The listing builds one solid part. Answer for the finished solid, in the listing's coordinates (mm). Face numbers are marked on the shaded views. A direction names the side the tool comes from. Round coordinates to 2 decimals unless told otherwise and drop trailing zeros. Order: outer loops, then holes, each group sorted by start corner. A loop starts at its lowest first (then second) coordinate and runs counter-clockwise, first axis right, second up. Notation, with made-up numbers: M 22,79.25 L 58,79.25 A27 cw 58,115.25 Z; hole C 82,-18.5 d3. An arc over 180 degrees is marked long. Write item = value, one per line. Start each with the question number.
(1) A cutting plane is placed at C-C, the plane z = 0. Determine the outline of the cut face in (x, y).
(2) A cutting plane is placed at B-B, the plane x = -14.5. Determine the outline of the cut face in (y, z), and give its area (3 significant figures).
(3) Each of these flat-tipped pins is pushed along its axis until it touches: pin 1 (1 mm diameter, centred on y = 17, z = -20, fed in from -X); pin 2 (4.5 mm diameter, centred on y = 8.69, z = -18.47, fed in from +X); pin 3 (3 mm diameter, centred on x = -17.5, y = 7, fed in from +Z). Where does it stop, or does it pass through?
(4) A cutting plane is placed at A-A, the plane z = -18. Determine the outline of the cut face in (x, y), and give its area (3 significant figures).
(5) Which of the six approach directions +Z, -Z, +X, -X, +Y, -Y give full straight-line access (tool end or side, diameter ignored) to the marked faces 4, 5, 6, 7 and 8?
(6) Straight lines are drawn through the part: probe 1 along X at (y, z) = (12.5, -13); probe 2 along X at (y, z) = (14.25, 15); probe 3 along Z at (x, y) = (0, 20). For each, find the intervals that lie inside material, in ascending order. Write a range as from..to.
(7) A cutting plane is placed at D-D, the plane x = 12.5. Determine the outline of the cut face in (y, z), and give its area (3 significant figures).
(8) For a pull along X with two mould halves and no side action, classify the marked faces 1, 2 and 3 as released by +X, released by -X, zero draft, split by the parting line, or undercut.
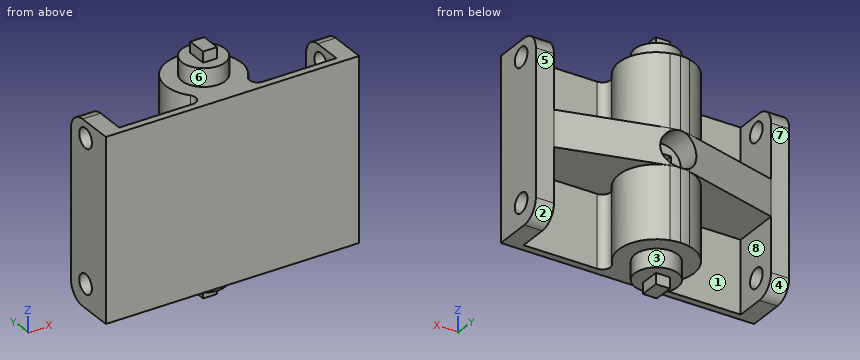
from build123d import *
from build123d.topology import SkipClean

# Parameters (mm, degrees)
BOSS_EXTRUDE1_DEPTH      = 5
BOSS_EXTRUDE2_DEPTH      = 20
MIRROR3_COPY_1_DEPTH     = 5
MIRROR3_COPY_2_DEPTH     = 20
SKETCH4_R                = 2.698355907
CUT_EXTRUDE1_DEPTH       = 5
BOSS_EXTRUDE3_DEPTH      = 5
BOSS_EXTRUDE3_DEPTH_BACK = 55
SKETCH8_R                = 5.951026126
SKETCH8_W                = 3.866122338
SKETCH8_H                = 5.532358837
BOSS_EXTRUDE5_DEPTH      = 3
BOSS_EXTRUDE5_DEPTH_BACK = 63
SKETCH10_W               = 3.866122338
SKETCH10_H               = 5.532358837
SKETCH12_R               = 5
CUT_EXTRUDE3_DEPTH       = 7.59683428
SKETCH14_W               = 4.609426796
SKETCH14_H               = 4.865506062
CUT_EXTRUDE6_DEPTH       = 4


with BuildPart() as part:
    # Sketch1 → Boss-Extrude1 (new body)
    with BuildSketch(Plane.XY):
        with BuildLine():
            Line((30, 2), (30, 15))
            Line((30, 15), (2.700298335, 22.368034529))
            ThreePointArc((2.700298335, 22.368034529), (9.883500212, 15.478856519), (7.950094011, 5.715603818))
            ThreePointArc((7.950094011, 5.715603818), (7.635951646, 3.305180914), (9.686640989, 2))
            Line((9.686640989, 2), (30, 2))
        make_face()
        with BuildLine():
            ThreePointArc((7.950094011, 5.715603818), (7.635951646, 3.305180914), (9.686640989, 2))
            Line((9.686640989, 2), (30, 2))
            Line((30, 2), (30, 15))
            Line((30, 15), (35, 15))
            Line((35, 15), (35, 0))
            Line((35, 0), (0, 0))
            Line((0, 0), (0, 2))
            Line((0, 2), (0, 6.411987573))
            ThreePointArc((0, 6.411987573), (5.951026126, 12.363013699), (0, 18.314039825))
            Line((0, 18.314039825), (0, 22.726027397))
            ThreePointArc((0, 22.726027397), (9.388270676, 16.750772424), (7.950094011, 5.715603818))
        make_face()
    boss_extrude1 = extrude(amount=BOSS_EXTRUDE1_DEPTH)

    # Sketch3 → Boss-Extrude2 (add)
    with BuildSketch(Plane.XY.offset(5)):
        with BuildLine():
            ThreePointArc((7.950094011, 5.715603818), (9.883500212, 15.478856519), (2.700298335, 22.368034529))
            ThreePointArc((2.700298335, 22.368034529), (1.361962737, 22.636139339), (0, 22.726027397))
            Line((0, 22.726027397), (0, 18.314039825))
            ThreePointArc((0, 18.314039825), (5.951026126, 12.363013699), (0, 6.411987573))
            Line((0, 6.411987573), (0, 2))
            Line((0, 2), (0, 0))
            Line((0, 0), (35, 0))
            Line((35, 0), (35, 15))
            Line((35, 15), (30, 15))
            Line((30, 15), (30, 2))
            Line((30, 2), (9.686640989, 2))
            ThreePointArc((9.686640989, 2), (7.635951646, 3.305180914), (7.950094011, 5.715603818))
        make_face()
    boss_extrude2 = extrude(amount=BOSS_EXTRUDE2_DEPTH)

    # Mirror2: Boss-Extrude1, Boss-Extrude2 across plane
    add(boss_extrude1.mirror(Plane.ZY))
    add(boss_extrude2.mirror(Plane.ZY))

    # Mirror3: Boss-Extrude1, Boss-Extrude2 across Front Plane
    with SkipClean():  # the faces are left unmerged after this step: merging them gives an invalid solid
        add(boss_extrude1.mirror(Plane.XY))
        add(boss_extrude2.mirror(Plane.XY))

    # Mirror3 copy 1 sketch → Mirror3 copy 1 (add)
    with BuildSketch(Plane(origin=(0, 0, 0), x_dir=(-1, 0, 0), z_dir=(0, 0, -1))):
        with BuildLine():
            Line((30, 2), (30, 15))
            Line((30, 15), (2.700298335, 22.368034529))
            ThreePointArc((2.700298335, 22.368034529), (9.883500212, 15.478856519), (7.950094011, 5.715603818))
            ThreePointArc((7.950094011, 5.715603818), (7.635951646, 3.305180914), (9.686640989, 2))
            Line((9.686640989, 2), (30, 2))
        make_face()
        with BuildLine():
            ThreePointArc((7.950094011, 5.715603818), (7.635951646, 3.305180914), (9.686640989, 2))
            Line((9.686640989, 2), (30, 2))
            Line((30, 2), (30, 15))
            Line((30, 15), (35, 15))
            Line((35, 15), (35, 0))
            Line((35, 0), (0, 0))
            Line((0, 0), (0, 2))
            Line((0, 2), (0, 6.411987573))
            ThreePointArc((0, 6.411987573), (5.951026126, 12.363013699), (0, 18.314039825))
            Line((0, 18.314039825), (0, 22.726027397))
            ThreePointArc((0, 22.726027397), (9.388270676, 16.750772424), (7.950094011, 5.715603818))
        make_face()
    extrude(amount=MIRROR3_COPY_1_DEPTH)

    # Mirror3 copy 2 sketch → Mirror3 copy 2 (add)
    with SkipClean():  # the faces are left unmerged after this step: merging them gives an invalid solid
        with BuildSketch(Plane(origin=(0, 0, -5), x_dir=(-1, 0, 0), z_dir=(0, 0, -1))):
            with BuildLine():
                ThreePointArc((7.950094011, 5.715603818), (9.883500212, 15.478856519), (2.700298335, 22.368034529))
                ThreePointArc((2.700298335, 22.368034529), (1.361962737, 22.636139339), (0, 22.726027397))
                Line((0, 22.726027397), (0, 18.314039825))
                ThreePointArc((0, 18.314039825), (5.951026126, 12.363013699), (0, 6.411987573))
                Line((0, 6.411987573), (0, 2))
                Line((0, 2), (0, 0))
                Line((0, 0), (35, 0))
                Line((35, 0), (35, 15))
                Line((35, 15), (30, 15))
                Line((30, 15), (30, 2))
                Line((30, 2), (9.686640989, 2))
                ThreePointArc((9.686640989, 2), (7.635951646, 3.305180914), (7.950094011, 5.715603818))
            make_face()
        extrude(amount=MIRROR3_COPY_2_DEPTH)

    # Sketch4 → Cut-Extrude1 (cut)
    with SkipClean():  # the faces are left unmerged after this step: merging them gives an invalid solid
        with BuildSketch(Plane(origin=(35, 0, 0), x_dir=(0, 0, -1), z_dir=(1, 0, 0))):
            with Locations((-20.507504892, 8.694639524)):
                Circle(SKETCH4_R)
            with Locations((18.468747096, 8.694639524)):
                Circle(SKETCH4_R)
            with BuildLine():
                Line((-25, 10), (-27.403303321, 11.153141573))
                Line((-27.403303321, 11.153141573), (-26.20165166, 17.389341891))
                Line((-26.20165166, 17.389341891), (-20, 16.194347401))
                Line((-20, 16.194347401), (-20, 15))
                ThreePointArc((-20, 15), (-23.535533906, 13.535533906), (-25, 10))
            make_face()
            with BuildLine():
                Line((20, 15), (20.74735875, 17.389341891))
                Line((20.74735875, 17.389341891), (31.360891984, 16.194670945))
                Line((31.360891984, 16.194670945), (27.103485998, 9.174347241))
                Line((27.103485998, 9.174347241), (25, 10))
                ThreePointArc((25, 10), (23.535533906, 13.535533906), (20, 15))
            make_face()
        cut_extrude1 = extrude(amount=-CUT_EXTRUDE1_DEPTH, mode=Mode.SUBTRACT)

    # Mirror4: Cut-Extrude1 across plane
    with SkipClean():  # the faces are left unmerged after this step: merging them gives an invalid solid
        add(cut_extrude1.mirror(Plane.ZY), mode=Mode.SUBTRACT)

    # Sketch8 → Boss-Extrude3 (add, two sides: drawn at the far end of the back side and taken through both)
    with SkipClean():  # the faces are left unmerged after this step: merging them gives an invalid solid
        with BuildSketch(Plane.XY.offset(25).offset(-BOSS_EXTRUDE3_DEPTH_BACK)):
            with Locations((0, 12.363013699)):
                Circle(SKETCH8_R)
            with Locations((0, 12.363013699)):
                Rectangle(SKETCH8_W, SKETCH8_H, mode=Mode.SUBTRACT)
        extrude(amount=BOSS_EXTRUDE3_DEPTH + BOSS_EXTRUDE3_DEPTH_BACK)

    # Sketch10 → Boss-Extrude5 (add, two sides: drawn at the far end of the back side and taken through both)
    with SkipClean():  # the faces are left unmerged after this step: merging them gives an invalid solid
        with BuildSketch(Plane.XY.offset(30).offset(-BOSS_EXTRUDE5_DEPTH_BACK)):
            with Locations((0, 12.363013699)):
                Rectangle(SKETCH10_W, SKETCH10_H)
        extrude(amount=BOSS_EXTRUDE5_DEPTH + BOSS_EXTRUDE5_DEPTH_BACK)

    # Sketch12 → Cut-Extrude3 (cut)
    with SkipClean():  # the faces are left unmerged after this step: merging them gives an invalid solid
        with BuildSketch(Plane.XZ.offset(-22.726027397)):
            with Locations(Location((0, 0, 0), (0, 0, 57.312299274))):
                Circle(SKETCH12_R)
        extrude(amount=CUT_EXTRUDE3_DEPTH, mode=Mode.SUBTRACT)

    # Sketch14 → Cut-Extrude6 (cut, symmetric)
    with SkipClean():  # the faces are left unmerged after this step: merging them gives an invalid solid
        with BuildSketch(Plane(origin=(0, 15.129193117, 0), x_dir=(1, 0, 0), z_dir=(0, 1, 0))):
            Rectangle(SKETCH14_W, SKETCH14_H)
        extrude(amount=CUT_EXTRUDE6_DEPTH, both=True, mode=Mode.SUBTRACT)


solid = part.part
Reported:
q1.outline = M -35,0 L 35,0 L 35,15 L 30,15 L 5,21.75 L 5,15.13 L 2.3,15.13 L 2.3,11.13 L -2.3,11.13 L -2.3,15.13 L -5,15.13 L -5,21.75 L -30,15 L -35,15 Z
q2.outline = M 0,-25 L 2,-25 L 2,-5 L 19.18,-5 L 19.18,5 L 2,5 L 2,25 L 0,25 Z
q2.area = 272 mm²
q3.pin_1 = -9.5
q3.pin_2 = 10.26
q3.pin_3 = 5
q4.outline = M -35,0 L 35,0 L 35,6.04 L 30,6.04 L 30,2 L 9.69,2 A2.26 cw 7.95,5.72 A10.36 ccw long -7.95,5.72 A2.26 cw -9.69,2 L -30,2 L -30,6.04 L -35,6.04 Z; M -35,11.35 L -30,11.35 L -30,15 L -35,15 Z; M 30,11.35 L 35,11.35 L 35,15 L 30,15 Z
q4.area = 571 mm²
q5.face_4 = -Z, -X, +Y
q5.face_5 = +Z, -Z, +X, +Y
q5.face_6 = +Z
q5.face_7 = +Z, -Z, -X, +Y
q5.face_8 = -Z, +Y
q6.probe_1 = -35..-30, -10.36..10.36, 30..35
q6.probe_2 = -35..-30, -10.19..10.19, 30..35
q6.probe_3 = -25..-5, 5..25
q7.outline = M 0,-25 L 2,-25 L 2,-5 L 19.72,-5 L 19.72,5 L 2,5 L 2,25 L 0,25 Z
q7.area = 277 mm²
q8.face_1 = undercut
q8.face_2 = zero draft
q8.face_3 = split by the parting line
